Verification items for this drawing (mm, ordinates from the low corner). A direction names the side the tool comes from. Round coordinates to 2 decimals unless told otherwise and drop trailing zeros. Order: outer loops, then holes, each group sorted by start corner. A loop starts at its lowest first (then second) coordinate and runs counter-clockwise, first axis right, second up. Notation, with made-up numbers: M -1,74.25 L 46,74.25 A19 ccw 46,90.25 Z; hole C 2.5,87 d11. An arc over 180 degrees is marked long. Use CSV: the item, a comma, the result in double quotes. Start each with the question number.
Q1. Set-up check for the marked faces 1, 2 and 3: record each of +Z, -Z, +X, -X, +Y, -Y from which the full face is reachable in a straight line by a thin tool's end or side.
Q2. Gauge pin test, flat ends, axial feed: pin 1 Ø6 at (y, z) = (13.5, 13) entering from -X; pin 2 Ø4 at (x, y) = (32, 13) entering from -Z; pin 3 Ø5 at (x, y) = (13, 14.5) entering from -Z; pin 4 Ø4 at (x, z) = (37, 11.5) entering from +Y. Record the tip position at first contact, or that the pin passes through.
Q3. Scan lines: line 1 (X direction, y = 7.25, z = 6); line 2 (X direction, y = 11.5, z = 18.75); line 3 (Y direction, x = 36, z = 10.25). Record each from-to range of solid material in increasing order.
Q4. Sectioned sample at A-A (z = 10). Enter the section's corners in (x, y).
Q5. Sectioned sample at B-B (x = 29.5). Enter the section's corners in (y, z).
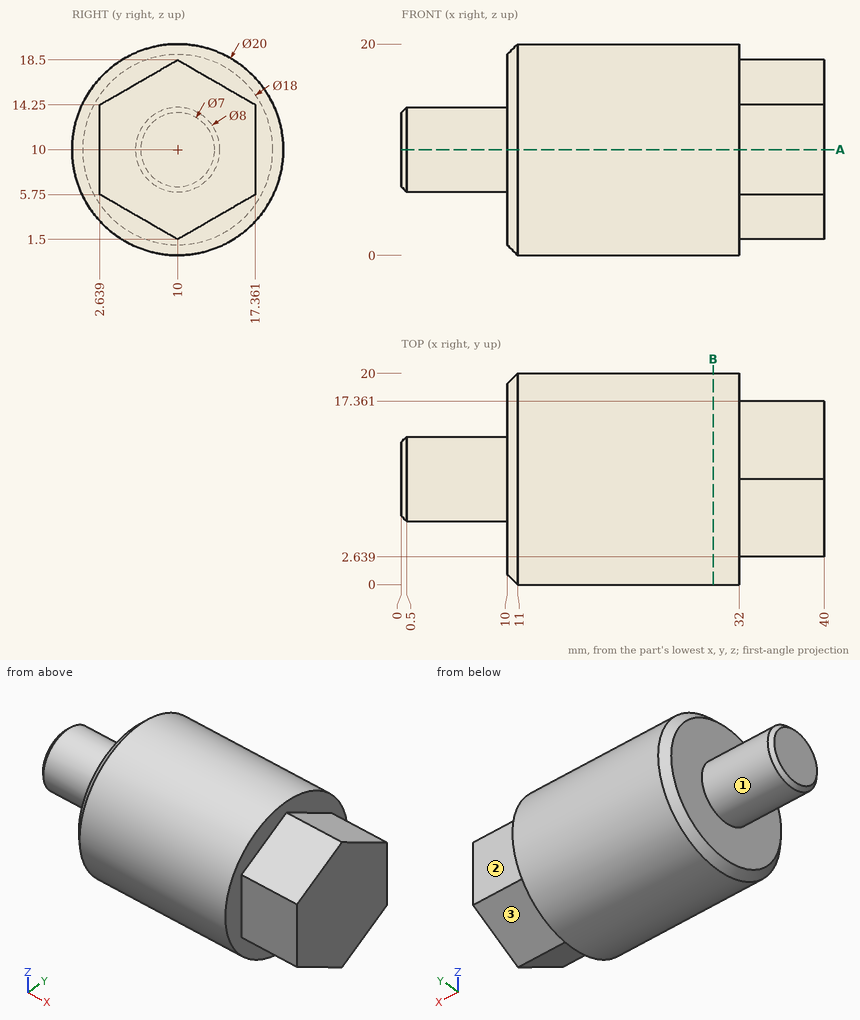
Verdict:
1,face 1,"-X"
1,face 2,"+Z, -Z, +X, +Y"
1,face 3,"-Z, +X, +Y"
2,pin 1,"stops at x = 0"
2,pin 2,"stops at z = 0.05"
2,pin 3,"stops at z = 0.2"
2,pin 4,"stops at y = 17.36"
3,line 1,"x = 10 to 40"
3,line 2,"x = 10 to 32"
3,line 3,"y = 2.64 to 17.36"
4,outline,"M 0,6.5 L 0.5,6 L 10,6 L 10,1 L 11,0 L 32,0 L 32,2.64 L 40,2.64 L 40,17.36 L 32,17.36 L 32,20 L 11,20 L 10,19 L 10,14 L 0.5,14 L 0,13.5 Z"
5,outline,"C 10,10 d20"
